from build123d import *

# Parameters (mm, degrees)
BOSS_EXTRUDE1_DEPTH    = 46.39999966
SKETCH2_R              = 1.3500000000000056
SKETCH2_R_2            = 1.3500000000000065
SKETCH2_R_3            = 1.3500000000000034
CUT_EXTRUDE1_DEPTH     = 57.705554564416346
CUT_EXTRUDE2_DEPTH     = 57.705554564416346
CUT_EXTRUDE3_DEPTH     = 77.91241719292147
MOVE_FACE1_BY          = 0.5
MOVE_FACE1_2_BY        = 0.5
CUT_EXTRUDE5_DEPTH     = 0.5
CUT_EXTRUDE6_DEPTH     = 0.5
MOVE_START             = 2.95
MOVE_FACE2_OUTLINE_W   = 4.200000000000003
MOVE_FACE2_OUTLINE_H   = 47.399999660000006
MOVE_FACE2_OUTLINE_R   = 1.35
MOVE_FACE2_DEPTH       = 2
MOVE_FACE3_BY          = 2
MOVE_FACE4_BY          = 0.1
MOVE_FACE4_2_BY        = 0.1
MOVE_FACE4_3_BY        = 0.1
MOVE_FACE4_4_BY        = 0.1
SKETCH14_W             = 31.645569847246712
SKETCH14_H             = 25
BOSS_EXTRUDE4_DEPTH    = 4
SKETCH15_R             = 2.0999999999999974
SKETCH15_R_2           = 2.100000000000001
CUT_EXTRUDE9_DEPTH     = 59.74664856924181
SKETCH16_R             = 3.599999999999999
SKETCH16_R_2           = 3.600000000000001
SKETCH16_R_3           = 3.5999999999999996
CUT_EXTRUDE10_DEPTH    = 4.2
MOVE_START_2           = -6
MOVE_FACE5_OUTLINE_W   = 60.00000000000001
MOVE_FACE5_OUTLINE_H   = 47.399999660000006
MOVE_FACE5_OUTLINE_R   = 1.35
MOVE_FACE5_OUTLINE_W_2 = 31.645569848
MOVE_FACE5_OUTLINE_H_2 = 25.000000000000004
MOVE_FACE5_DEPTH       = 4
MOVE_FACE6_OUTLINE_W   = 60.00000000000001
MOVE_FACE6_OUTLINE_H   = 47.399999660000006
MOVE_FACE6_OUTLINE_R   = 1.35
MOVE_FACE6_OUTLINE_R_2 = 2.1
MOVE_FACE6_DEPTH       = 1
FILLET1_R              = 1
SKETCH18_W             = 20
SKETCH18_H             = 1
BOSS_EXTRUDE5_DEPTH    = 20
CHAMFER1_SIZE          = 0.5


# Read off the part's stored shape, not the designer's step: Move Face2, Move Face5, Move Face6
with BuildPart() as part:
    # Sketch1 → Boss-Extrude1 (new body)
    with BuildSketch(Plane.XY):
        Polygon((0, 0), (30.000000000000004, 0), (30.000000000000004, 12.749899999999984), (22.300099999999997, 12.749899999999984), (22.300099999999997, 9.749899999999984), (26, 6.050000000000002), (26, 4.950000000000001), (22.3, 4.95), (22.3, 1), (0, 1), align=None)
    extrude(amount=-BOSS_EXTRUDE1_DEPTH)

    # Mirror1: part across plane


with BuildPart() as part_1:
    add(part.part)
    add(part.part.mirror(Plane(origin=(0, 1, -46.39999966), x_dir=(0, 0, 1), z_dir=(-1, 0, 0))))

    # Sketch2 → Cut-Extrude1 (cut, through all)
    with BuildSketch(Plane(origin=(0, 12.749899999999984, 0), x_dir=(1, 0, 0), z_dir=(0, 1, 0))):
        with Locations(Location((-24.54999983142516, 1.9999999985748345, 0), (0, 0, 270))):
            Circle(SKETCH2_R)
        with Locations(Location((-24.54999983142517, 44.39999966142516, 0), (0, 0, 270))):
            Circle(SKETCH2_R_2)
        with Locations(Location((24.54999983142517, 1.9999999985748345, 0), (0, 0, 270))):
            Circle(SKETCH2_R)
        with Locations(Location((24.54999983142515, 44.39999966142516, 0), (0, 0, 270))):
            Circle(SKETCH2_R_3)
    extrude(amount=-CUT_EXTRUDE1_DEPTH, mode=Mode.SUBTRACT)

    # Sketch3 → Cut-Extrude2 (cut, through all)
    with BuildSketch(Plane.XY):
        Polygon((26.300000000000004, 12.749899999999984), (30.000000000000004, 9.049899999999985), (30.000000000000004, 12.749899999999984), align=None)
        Polygon((-30.000000000000004, 12.749899999999984), (-30.000000000000004, 9.049899999999981), (-26.300000000000004, 12.749899999999984), align=None)
    extrude(amount=-CUT_EXTRUDE2_DEPTH, mode=Mode.SUBTRACT)

    # Sketch4 → Cut-Extrude3 (cut, through all)
    with BuildSketch(Plane(origin=(30.000000000000004, 0, 0), x_dir=(0, 0, -1), z_dir=(1, 0, 0))):
        Polygon((9.199999829999998, 12.749899999999986), (37.199999829999996, 12.749899999999997), (30.41619190204875, 1.0000000000000036), (15.983807757951256, 0.9999999999999983), align=None)
    extrude(amount=-CUT_EXTRUDE3_DEPTH, mode=Mode.SUBTRACT)

    # Move Face1: a face moved outward by 0.5
    extrude(part_1.faces().sort_by_distance((-24, 3.187475, -46.39999966))[0], amount=MOVE_FACE1_BY, dir=(0, 0, -1))

    # Move Face1 2: a face moved outward by 0.5
    extrude(part_1.faces().sort_by_distance((-24, 3.187475, 0))[0], amount=MOVE_FACE1_2_BY, dir=(0, 0, 1))

    # Sketch6 → Cut-Extrude5 (cut)
    with BuildSketch(Plane(origin=(-26, 0, 0), x_dir=(0, 0, -1), z_dir=(1, 0, 0))):
        Polygon((13.703274194652213, 4.950000000000001), (13.068188898543607, 6.050000000000002), (-0.5000000000000004, 6.050000000000002), (-0.5000000000000004, 4.950000000000001), align=None)
        Polygon((33.33181076145639, 6.050000000000002), (32.69672546534779, 4.950000000000002), (46.89999966, 4.950000000000001), (46.89999966, 6.050000000000002), align=None)
    extrude(amount=-CUT_EXTRUDE5_DEPTH, mode=Mode.SUBTRACT)

    # Sketch7 → Cut-Extrude6 (cut)
    with BuildSketch(Plane.ZY.offset(-26)):
        Polygon((-13.068188898543607, 6.050000000000002), (-13.703274194652213, 4.950000000000001), (0.5000000000000004, 4.950000000000001), (0.5000000000000004, 6.050000000000002), align=None)
        Polygon((-32.69672546534779, 4.950000000000002), (-33.33181076145639, 6.050000000000002), (-46.89999966, 6.050000000000002), (-46.89999966, 4.950000000000001), align=None)
    extrude(amount=-CUT_EXTRUDE6_DEPTH, mode=Mode.SUBTRACT)

    # Move Face2 outline → Move Face2 (cut)
    # profile 1 of 2: a face of its own
    with BuildSketch(Plane(origin=(0, 0, 0), x_dir=(1, 0, 0), z_dir=(0, 1, 0)).offset(MOVE_START)):
        with Locations((-24.400000000000002, 23.199999830000003)):
            Rectangle(MOVE_FACE2_OUTLINE_W, MOVE_FACE2_OUTLINE_H)
        with Locations((-24.549999831, 1.999999999)):
            Circle(MOVE_FACE2_OUTLINE_R, mode=Mode.SUBTRACT)
        with Locations((-24.549999831, 44.399999661)):
            Circle(MOVE_FACE2_OUTLINE_R, mode=Mode.SUBTRACT)
    # profile 2 of 2: a face of its own
    with BuildSketch(Plane(origin=(0, 0, 0), x_dir=(1, 0, 0), z_dir=(0, 1, 0)).offset(MOVE_START)):
        with Locations((24.400000000000002, 23.199999830000003)):
            Rectangle(MOVE_FACE2_OUTLINE_W, MOVE_FACE2_OUTLINE_H)
        with Locations((24.549999831, 1.999999999)):
            Circle(MOVE_FACE2_OUTLINE_R, mode=Mode.SUBTRACT)
        with Locations((24.549999831, 44.399999661)):
            Circle(MOVE_FACE2_OUTLINE_R, mode=Mode.SUBTRACT)
    extrude(amount=MOVE_FACE2_DEPTH, mode=Mode.SUBTRACT)

    # Move Face3: a face moved outward by 2.0
    extrude(part_1.faces().sort_by_distance((0, 0, -23.19999983))[0], amount=MOVE_FACE3_BY, dir=(0, -1, 0))

    # Move Face4: a face moved inward by 0.1
    extrude(part_1.faces().sort_by_distance((-26.5, 4.468031617, -6.740769385))[0], amount=MOVE_FACE4_BY, dir=(-1, 0, 0), mode=Mode.SUBTRACT)

    # Move Face4 2: a face moved inward by 0.1
    extrude(part_1.faces().sort_by_distance((-26.5, 4.468031617, -39.659230275))[0], amount=MOVE_FACE4_2_BY, dir=(-1, 0, 0), mode=Mode.SUBTRACT)

    # Move Face4 3: a face moved inward by 0.1
    extrude(part_1.faces().sort_by_distance((26.5, 4.468031617, -6.740769385))[0], amount=MOVE_FACE4_3_BY, dir=(1, 0, 0), mode=Mode.SUBTRACT)

    # Move Face4 4: a face moved inward by 0.1
    extrude(part_1.faces().sort_by_distance((26.5, 4.468031617, -39.659230275))[0], amount=MOVE_FACE4_4_BY, dir=(1, 0, 0), mode=Mode.SUBTRACT)

    # Sketch14 → Boss-Extrude4 (add)
    with BuildSketch(Plane.XZ.offset(1.9999999999999996)):
        with Locations((-1.78e-15, -23.199999829999996)):
            Rectangle(SKETCH14_W, SKETCH14_H)
    extrude(amount=BOSS_EXTRUDE4_DEPTH)

    # Sketch15 → Cut-Extrude9 (cut, through all)
    with BuildSketch(Plane.XZ.offset(6)):
        with Locations(Location((-8.5, -14.699999829999992, 0), (0, 0, 270))):
            Circle(SKETCH15_R)
        with Locations(Location((8.5, -14.699999829999992, 0), (0, 0, 270))):
            Circle(SKETCH15_R)
        with Locations(Location((8.500000000000002, -31.699999829999992, 0), (0, 0, 270))):
            Circle(SKETCH15_R_2)
        with Locations(Location((-8.500000000000002, -31.699999829999992, 0), (0, 0, 270))):
            Circle(SKETCH15_R_2)
    extrude(amount=-CUT_EXTRUDE9_DEPTH, mode=Mode.SUBTRACT)

    # Sketch16 → Cut-Extrude10 (cut)
    with BuildSketch(Plane(origin=(0, 1, 0), x_dir=(1, 0, 0), z_dir=(0, 1, 0))):
        with Locations(Location((-8.500000000000002, 31.699999829999992, 0), (0, 0, 270))):
            Circle(SKETCH16_R)
        with Locations(Location((8.500000000000002, 31.699999829999992, 0), (0, 0, 270))):
            Circle(SKETCH16_R_2)
        with Locations(Location((8.5, 14.699999829999992, 0), (0, 0, 270))):
            Circle(SKETCH16_R_3)
        with Locations(Location((-8.5, 14.699999829999992, 0), (0, 0, 270))):
            Circle(SKETCH16_R_3)
    extrude(amount=-CUT_EXTRUDE10_DEPTH, mode=Mode.SUBTRACT)

    # Move Face5 outline → Move Face5 (add)
    with BuildSketch(Plane(origin=(0, 0, 0), x_dir=(1, 0, 0), z_dir=(0, 1, 0)).offset(MOVE_START_2)):
        with Locations((0, 23.199999830000003)):
            Rectangle(MOVE_FACE5_OUTLINE_W, MOVE_FACE5_OUTLINE_H)
        with Locations((-24.549999831, 1.999999999)):
            Circle(MOVE_FACE5_OUTLINE_R, mode=Mode.SUBTRACT)
        with Locations((24.549999831, 1.999999999)):
            Circle(MOVE_FACE5_OUTLINE_R, mode=Mode.SUBTRACT)
        with Locations((-24.549999831, 44.399999661)):
            Circle(MOVE_FACE5_OUTLINE_R, mode=Mode.SUBTRACT)
        with Locations((0, 23.199999830000003)):
            Rectangle(MOVE_FACE5_OUTLINE_W_2, MOVE_FACE5_OUTLINE_H_2, mode=Mode.SUBTRACT)
        with Locations((24.549999831, 44.399999661)):
            Circle(MOVE_FACE5_OUTLINE_R, mode=Mode.SUBTRACT)
    extrude(amount=MOVE_FACE5_DEPTH)

    # Move Face6 outline → Move Face6 (cut)
    with BuildSketch(Plane(origin=(0, 0, 0), x_dir=(1, 0, 0), z_dir=(0, 1, 0)).offset(MOVE_START_2)):
        with Locations((0, 23.199999830000003)):
            Rectangle(MOVE_FACE6_OUTLINE_W, MOVE_FACE6_OUTLINE_H)
        with Locations((-24.549999831, 1.999999999)):
            Circle(MOVE_FACE6_OUTLINE_R, mode=Mode.SUBTRACT)
        with Locations((-8.5, 14.69999983)):
            Circle(MOVE_FACE6_OUTLINE_R_2, mode=Mode.SUBTRACT)
        with Locations((24.549999831, 1.999999999)):
            Circle(MOVE_FACE6_OUTLINE_R, mode=Mode.SUBTRACT)
        with Locations((8.5, 14.69999983)):
            Circle(MOVE_FACE6_OUTLINE_R_2, mode=Mode.SUBTRACT)
        with Locations((-8.5, 31.69999983)):
            Circle(MOVE_FACE6_OUTLINE_R_2, mode=Mode.SUBTRACT)
        with Locations((-24.549999831, 44.399999661)):
            Circle(MOVE_FACE6_OUTLINE_R, mode=Mode.SUBTRACT)
        with Locations((8.5, 31.69999983)):
            Circle(MOVE_FACE6_OUTLINE_R_2, mode=Mode.SUBTRACT)
        with Locations((24.549999831, 44.399999661)):
            Circle(MOVE_FACE6_OUTLINE_R, mode=Mode.SUBTRACT)
    extrude(amount=MOVE_FACE6_DEPTH, mode=Mode.SUBTRACT)

    # Fillet1
    fillet1_edges = [part_1.edges().sort_by_distance(p)[0] for p in [
        (30.000000000000004, 2.0249499999999934, -46.89999966),
        (30.000000000000004, 2.0249499999999934, 0.5),
        (-30.000000000000004, 2.0249499999999907, 0.5),
        (-30.000000000000004, 2.02494999999999, -46.89999966),
        (28.150000000000006, 10.899899999999985, -46.899999660000006),
        (28.150000000000006, 10.899899999999985, 0.5),
        (-28.150000000000006, 10.899899999999983, -46.899999660000006),
        (-28.150000000000006, 10.899899999999983, 0.5),
    ]]
    fillet(fillet1_edges, radius=FILLET1_R)

    # Sketch18 → Boss-Extrude5 (add)
    with BuildSketch(Plane.XY.offset(0.5)):
        with Locations((0, -4.499999999999998)):
            Rectangle(SKETCH18_W, SKETCH18_H)
    extrude(amount=BOSS_EXTRUDE5_DEPTH)

    # Chamfer1
    chamfer1_edges = [part_1.edges().sort_by_distance(p)[0] for p in [
        (30, -5, -23.19999983),
        (0, -5, -46.89999966),
        (-19.5, -5, 0.5),
        (-30, -5, -23.19999983),
        (-29.707106781186546, -5, -46.607106441186545),
        (-29.707106781186543, -5, 0.20710678118654768),
        (29.707106781186546, -5, 0.20710678118654768),
        (29.707106781186546, -5, -46.607106441186545),
        (-10, -4.999999999999998, 10.5),
        (10, -4.999999999999998, 10.5),
        (0, -4.999999999999998, 20.5),
    ]]
    chamfer(chamfer1_edges, length=CHAMFER1_SIZE)


solid = part_1.part
CAD build for the part. Positions are in the model's coordinates, mm. A direction names the side the tool comes from. Give positions to 0.01 mm unless a question says otherwise; leave off trailing zeros. Order: outer loops, then holes, each group sorted by start corner. A loop starts at its lowest first (then second) coordinate and runs counter-clockwise, first axis right, second up. Notation, with made-up numbers: (17.25, -16.75) -> (27.25, -16.75) arc R18 ccw to (27.25, 17.25) -> close; hole circle Ø6 at (56.25, -0.5). An arc over 180 degrees is marked (long way). Return JSON: item names as keys, results as strings.
Q1. Saw through at B-B (y = -1). Count the separate pieces of the cut face and the enclosed holes in it, then the cut area to 3 significant figures.
Working result:
{"separate pieces": "1", "enclosed holes": "8", "area": "2,660 mm²"}
Q2. Which spindle directions (+Z, -Z, +X, -X, +Y, -Y) get a long thin tool onto all of the face, cutting with end or side? Do faces 5 (the face through (26.6, 5, -39)), 6 (the face through (-22.3, 11, -5)), 7 (the face through (-4.93, -1.07, -32.17)), 8 (the face through (0, -4, 10)). Say none if no direction does.
Working result:
{"face 5": "+Z, -Z", "face 6": "+Z, -Z, +Y", "face 7": "+Y", "face 8": "+Z, +X, -X, +Y"}
Q3. Mould opens along Y. For faces 1 (the face through (-25.75, 10.23, -1.38)), 2 (the face through (26.6, 5, -7)), 3 (the face through (-24, 12.75, -4)), 4 (the face through (0, -5, -21)) say: pulls with the +Y half, pulls with the -Y half, needs draft (parallel to the pull), parting line crosses it, or undercut.
Working result:
{"face 1": "needs draft", "face 2": "undercut", "face 3": "pulls with the +Y half", "face 4": "pulls with the -Y half"}
Q4. Drill centre lines: line 1 (X direction, y = -0.35, z = -31.7); line 2 (Z direction, x = -24.55, y = -3.4); line 3 (X direction, y = -3.7, z = -14.7). Where is each one in solid material? Low to high.
Working result:
{"line 1": "-30 to -12.1, -4.9 to 4.9, 12.1 to 30", "line 2": "-46.9 to -45.75, -43.05 to -3.35, -0.65 to 0.5", "line 3": "-30 to -10.6, -6.4 to 6.4, 10.6 to 30"}
Q5. Flat gauge pins, fed straight in: pin 1 (2 mm diameter, centred on x = 8, z = -40, fed in from +Y); pin 2 (0.9 mm diameter, centred on y = 11, z = -3, fed in from +X); pin 3 (2.5 mm diameter, centred on y = 10.5, z = -42, fed in from +X). Where does each tip first touch, or does it go through?
Working result:
{"pin 1": "y = 1", "pin 2": "x = 28.5", "pin 3": "x = 29.8"}
Q6. Saw through at A-A (x = -8.5). Write the cut outline in (y, z), then the cut area to 3 significant figures.
Working result:
{"outline": "(-5, -46.4) -> (-4.5, -46.9) -> (1, -46.9) -> (1, -35.3) -> (-3.2, -35.3) -> (-3.2, -33.8) -> (-5, -33.8) -> close; (-5, -29.6) -> (-3.2, -29.6) -> (-3.2, -28.1) -> (1, -28.1) -> (1, -18.3) -> (-3.2, -18.3) -> (-3.2, -16.8) -> (-5, -16.8) -> close; (-5, -12.6) -> (-3.2, -12.6) -> (-3.2, -11.1) -> (1, -11.1) -> (1, 0.5) -> (-4, 0.5) -> (-4, 20.5) -> (-4.5, 20.5) -> (-5, 20) -> close", "area": "229 mm²"}
